Geometry check sheet. Reference: the model listing, model coordinates, mm. Coordinates: 2 decimals unless noted, no trailing zeros. Write each loop counter-clockwise with the first axis right and the second up, starting at its lowest first coordinate (ties: lowest second). Pieces come first, ordered by that corner, then holes. Notation, with made-up numbers: (-38, 19.25) - (-23, 19.25) arc R12 cw to (-23, 25.25) - close; hole circle Ø8 at (73, 5.5). An arc over 180 degrees is marked (long way). Answer as a JSON object with one key per item and string values. Group by question number.
from build123d import *

# Parameters (mm, degrees)
SKETCH_3_R          = 6.55
EXTRUDE_1_DEPTH     = 1.5
CUT_EXTRUDE_3_DEPTH = 346.626566427
EXTRUDE_2_DEPTH     = 3
CHAMFER_1_SIZE      = 4
SKETCH_8_R          = 1
SKETCH_8_R_2        = 1.6
CUT_EXTRUDE_6_DEPTH = 345.981177834
SKETCH_9_R          = 1.1
SKETCH_9_R_2        = 1.6
CUT_EXTRUDE_7_DEPTH = 345.981177834
CUT_EXTRUDE_8_DEPTH = 345.981177834
FILLET_4_R          = 50
FILLET_5_R          = 3
FILLET_6_R          = 1
EXTRUDE_3_DEPTH     = 3


with BuildPart() as part:
    # 草图3 → 凸台-拉伸1 (new, symmetric)
    # profile 1 of 2: a face of its own
    with BuildSketch(Plane(origin=(0, 0, 0), x_dir=(1, 0, 0), z_dir=(0, 1, 0))):
        with BuildLine():
            ThreePointArc((11.046281859, 5.956690113), (-6.46534327, 44.807884696), (-18.295362458, 85.748365655))
            Line((-18.295362458, 85.748365655), (-41.732882117, 195.59746049))
            Line((-41.732882117, 195.59746049), (-24.830239517, 252.12165071))
            ThreePointArc((-24.830239517, 252.12165071), (4.01455016, 296.880361934), (52.313928116, 319.29763677))
            Line((52.313928116, 319.29763677), (49.5768988, 337.088327327))
            ThreePointArc((49.5768988, 337.088327327), (-8.975981148, 310.878563044), (-45.908014731, 258.424617632))
            Line((-45.908014731, 258.424617632), (-76.290123868, 173.944647702))
            Line((-76.290123868, 173.944647702), (-14.508857835, 4.202014333))
            ThreePointArc((-14.508857835, 4.202014333), (-13.227629582, 0.452324895), (-12.09596095, -3.34517992))
            ThreePointArc((-12.09596095, -3.34517992), (-4.680454366, 11.644562977), (11.046281859, 5.956690113))
        make_face()
    # profile 2 of 2: a face of its own
    with BuildSketch(Plane(origin=(0, 0, 0), x_dir=(1, 0, 0), z_dir=(0, 1, 0))):
        with BuildLine():
            ThreePointArc((12.09596095, -3.34517992), (8.478119914, -30), (12.09596095, -56.65482008))
            ThreePointArc((12.09596095, -56.65482008), (0, -72.55), (-12.09596095, -56.65482008))
            ThreePointArc((-12.09596095, -56.65482008), (-8.478119914, -30), (-12.09596095, -3.34517992))
            ThreePointArc((-12.09596095, -3.34517992), (0, 12.55), (12.09596095, -3.34517992))
        make_face()
        with Locations(Location((0, 0, 0), (0, 0, 270))):
            Circle(SKETCH_3_R, mode=Mode.SUBTRACT)
        with Locations(Location((0, -60, 0), (0, 0, 270))):
            Circle(SKETCH_3_R, mode=Mode.SUBTRACT)
    extrude(amount=EXTRUDE_1_DEPTH, both=True)

    # 草图7 → 切除-拉伸3 (cut, through all)
    with BuildSketch(Plane(origin=(0, 1.5, 0), x_dir=(1, 0, 0), z_dir=(0, 1, 0))):
        with BuildLine():
            Line((4.497487802, -34.493479197), (8.909760465, -39.281260509))
            ThreePointArc((8.909760465, -39.281260509), (8.493926314, -31.777928612), (8.642731975, -24.264556235))
            ThreePointArc((8.642731975, -24.264556235), (7.765481215, -25.952185157), (5.921402859, -26.418055622))
            ThreePointArc((5.921402859, -26.418055622), (1.171733543, -29.743809881), (4.497487802, -34.493479197))
        make_face()
    extrude(amount=-CUT_EXTRUDE_3_DEPTH, mode=Mode.SUBTRACT)

    # 草图7<3> → 凸台-拉伸2 (add)
    with BuildSketch(Plane(origin=(0, 1.5, 0), x_dir=(1, 0, 0), z_dir=(0, 1, 0))):
        with BuildLine():
            ThreePointArc((-8.909760465, -39.281260509), (-8.493926314, -31.777928612), (-8.642731975, -24.264556235))
            ThreePointArc((-8.642731975, -24.264556235), (-8.806680236, -25.524578384), (-9.419131852, -26.637878822))
            ThreePointArc((-9.419131852, -26.637878822), (-10.758632644, -29.837669281), (-10.103316411, -33.24405769))
            ThreePointArc((-10.103316411, -33.24405769), (-9.068630527, -36.176084637), (-8.909760465, -39.281260509))
        make_face()
    extrude(amount=-EXTRUDE_2_DEPTH)

    # 倒角1
    # the kernel refuses this chamfer: 4 mm, written as the material it takes off along each edge
    with BuildSketch(Plane(origin=(49.5768988, -11.786731952, -337.088327327), x_dir=(-0.9857681497508005, 0, 0.16811054380045146), z_dir=(0, 1, 0))) as chamfer_1_piece_1:
        with BuildLine():
            Line((3.936502909, 0), (CHAMFER_1_SIZE * 0.0162625743907, CHAMFER_1_SIZE * 0.999867755593))
            Line((CHAMFER_1_SIZE * 0.0162625743907, CHAMFER_1_SIZE * 0.999867755593), (0, 0))
            ThreePointArc((0, 0), (2.023873499, -0.015992695), (3.936502909, 0))
        make_face()
    extrude(amount=23.573463904, mode=Mode.SUBTRACT)
    with BuildSketch(Plane(origin=(52.313928116, -12.013080834, -319.29763677), x_dir=(-0.15205718425393844, 0, -0.9883716976506176), z_dir=(0, 1, 0))) as chamfer_1_piece_2:
        with BuildLine():
            Line((CHAMFER_1_SIZE, 0), (-0.087315026, 4.087315025))
            ThreePointArc((-0.087315026, 4.087315025), (-0.023083391, 2.101920628), (0, 0))
            Line((0, 0), (CHAMFER_1_SIZE, 0))
        make_face()
    extrude(amount=24.026161669, mode=Mode.SUBTRACT)

    # 草图8 → 切除-拉伸6 (cut, through all)
    with BuildSketch(Plane(origin=(0, 1.5, 0), x_dir=(1, 0, 0), z_dir=(0, 1, 0))):
        with Locations((37.433203796, 321.978777823)):
            Circle(SKETCH_8_R)
        with Locations((36.505654972, 328.007845179)):
            Circle(SKETCH_8_R)
        with Locations((33.1451912, 327.490850752)):
            Circle(SKETCH_8_R)
        with Locations((34.072740024, 321.461783396)):
            Circle(SKETCH_8_R)
        with Locations(Location((44.787418503, 332.089831456, 0), (0, 0, 270))):
            Circle(SKETCH_8_R_2)
        with Locations(Location((44.787418503, 322.089831456, 0), (0, 0, 270))):
            Circle(SKETCH_8_R_2)
        with Locations((-39.768291207, 258.363013678)):
            Circle(SKETCH_8_R)
        with Locations((-40.742386095, 255.105539327)):
            Circle(SKETCH_8_R)
        with Locations((-30.091676222, 255.469378864)):
            Circle(SKETCH_8_R)
        with Locations((-31.06577111, 252.211904513)):
            Circle(SKETCH_8_R)
        with Locations((-67.294758965, 181.587091045)):
            Circle(SKETCH_8_R)
        with Locations((-65.489494047, 178.705942216)):
            Circle(SKETCH_8_R)
        with Locations((-51.956878434, 191.197471934)):
            Circle(SKETCH_8_R)
        with Locations((-50.151613516, 188.316323105)):
            Circle(SKETCH_8_R)
        with Locations((-25.036284897, 88.28804372)):
            Circle(SKETCH_8_R)
        with Locations((-25.450272298, 84.913341595)):
            Circle(SKETCH_8_R)
        with Locations((-39.031373121, 90.004873825)):
            Circle(SKETCH_8_R)
        with Locations((-39.445360522, 86.6301717)):
            Circle(SKETCH_8_R)
        Polygon((36.353597787, 328.996216876), (37.58526098, 320.990406125), (34.224797208, 320.473411699), (32.993134015, 328.47922245), align=None)
        Polygon((-40.726371898, 258.649512175), (-29.133595531, 255.182880368), (-30.107690419, 251.925406016), (-41.700466786, 255.392037824), align=None)
        Polygon((-68.142155679, 181.056130775), (-51.10948172, 191.728432204), (-49.304216802, 188.847283375), (-66.336890761, 178.174981946), align=None)
        Polygon((-40.02393257, 90.126634825), (-24.043725449, 88.16628272), (-24.45771285, 84.791580595), (-40.437919971, 86.7519327), align=None)
    extrude(amount=-CUT_EXTRUDE_6_DEPTH, mode=Mode.SUBTRACT)

    # 草图9 → 切除-拉伸7 (cut, through all)
    with BuildSketch(Plane(origin=(0, 1.5, 0), x_dir=(1, 0, 0), z_dir=(0, 1, 0))):
        with Locations(Location((-30.569466556, 243.400339284, 0), (0, 0, 270))):
            Circle(SKETCH_9_R)
        with Locations(Location((25.150787489, 314.162258091, 0), (0, 0, 270))):
            Circle(SKETCH_9_R)
        with Locations(Location((10.249770173, 305.559151733, 0), (0, 0, 270))):
            Circle(SKETCH_9_R)
        with Locations(Location((-34.866944003, 229.02912891, 0), (0, 0, 270))):
            Circle(SKETCH_9_R)
        with Locations(Location((-2.930953467, 294.499211388, 0), (0, 0, 270))):
            Circle(SKETCH_9_R)
        with Locations(Location((-39.16442145, 214.657918537, 0), (0, 0, 270))):
            Circle(SKETCH_9_R)
        with Locations(Location((-40.493555813, 175.411721209, 0), (0, 0, 270))):
            Circle(SKETCH_9_R)
        with Locations(Location((-37.363589654, 160.741911673, 0), (0, 0, 270))):
            Circle(SKETCH_9_R)
        with Locations(Location((-33.190301442, 141.182165624, 0), (0, 0, 270))):
            Circle(SKETCH_9_R)
        with Locations(Location((-33.646848365, 128, 0), (0, 0, 270))):
            Circle(SKETCH_9_R_2)
        with Locations(Location((-25.254946433, 99.197639299, 0), (0, 0, 270))):
            Circle(SKETCH_9_R_2)
        with Locations(Location((-37.131526919, 111.360979134, 0), (0, 0, 270))):
            Circle(SKETCH_9_R_2)
    extrude(amount=-CUT_EXTRUDE_7_DEPTH, mode=Mode.SUBTRACT)

    # 草图10 → 切除-拉伸8 (cut, through all)
    with BuildSketch(Plane(origin=(0, 1.5, 0), x_dir=(1, 0, 0), z_dir=(0, 1, 0))):
        Polygon((-42.197304508, 245.103074872), (-59.836896552, 196.054728732), (-47.97334255, 203.488172514), align=None)
        Polygon((-64.127048511, 169.764916812), (-48.531264313, 179.536894505), (-38.537074534, 132.695218557), (-48.388180029, 126.522731048), align=None)
    extrude(amount=-CUT_EXTRUDE_8_DEPTH, mode=Mode.SUBTRACT)

    # 圆角4
    fillet_4_edges = [part.edges().sort_by_distance(p)[0] for p in [
        (-41.732882117, 0, -195.59746049),
        (-76.290123868, 0, -173.944647702),
    ]]
    fillet(fillet_4_edges, radius=FILLET_4_R)

    # 圆角5
    fillet_5_edges = [part.edges().sort_by_distance(p)[0] for p in [
        (-48.388180029, 0, -126.522731048),
        (-64.127048511, 0, -169.764916812),
        (-48.531264313, 0, -179.536894505),
        (-38.537074534, 0, -132.695218557),
        (4.497487802, 0, 34.493479197),
        (8.909760465, 0, 39.281260509),
    ]]
    fillet(fillet_5_edges, radius=FILLET_5_R)

    # 圆角6
    fillet_6_edges = [part.edges().sort_by_distance(p)[0] for p in [
        (-42.197304508, 0, -245.103074872),
        (-47.97334255, 0, -203.488172514),
        (-59.836896552, 0, -196.054728732),
    ]]
    fillet(fillet_6_edges, radius=FILLET_6_R)

    # 草图11 → 凸台-拉伸3 (add)
    with BuildSketch(Plane(origin=(0, 1.5, 0), x_dir=(1, 0, 0), z_dir=(0, 1, 0))):
        with BuildLine():
            ThreePointArc((3.862363202, -34.328152946), (4.521977485, -34.653012522), (5.082760511, -35.12856183))
            Line((5.082760511, -35.12856183), (5.760441827, -35.863917549))
            ThreePointArc((5.760441827, -35.863917549), (4.207468493, -30.616888071), (7.413296366, -26.182284124))
            ThreePointArc((7.413296366, -26.182284124), (6.687056269, -26.42486787), (5.921402859, -26.418055622))
            ThreePointArc((5.921402859, -26.418055622), (1.241668153, -29.422934282), (3.862363202, -34.328152946))
        make_face()
        with BuildLine():
            Line((-14.508857835, 4.202014333), (-42.305901268, 80.573763491))
            ThreePointArc((-42.305901268, 80.573763491), (-22.483207982, 11.333558383), (-12.55, -60))
            ThreePointArc((-12.55, -60), (-12.435972216, -58.312073746), (-12.09596095, -56.65482008))
            ThreePointArc((-12.09596095, -56.65482008), (-10.118516623, -48.038526559), (-8.909760465, -39.281260509))
            ThreePointArc((-8.909760465, -39.281260509), (-9.068630527, -36.176084637), (-10.103316411, -33.24405769))
            ThreePointArc((-10.103316411, -33.24405769), (-10.758632644, -29.837669281), (-9.419131852, -26.637878822))
            ThreePointArc((-9.419131852, -26.637878822), (-8.806680236, -25.524578384), (-8.642731975, -24.264556235))
            ThreePointArc((-8.642731975, -24.264556235), (-10.536060501, -9.817012165), (-14.508857835, 4.202014333))
        make_face()
    extrude(amount=-EXTRUDE_3_DEPTH)


solid = part.part
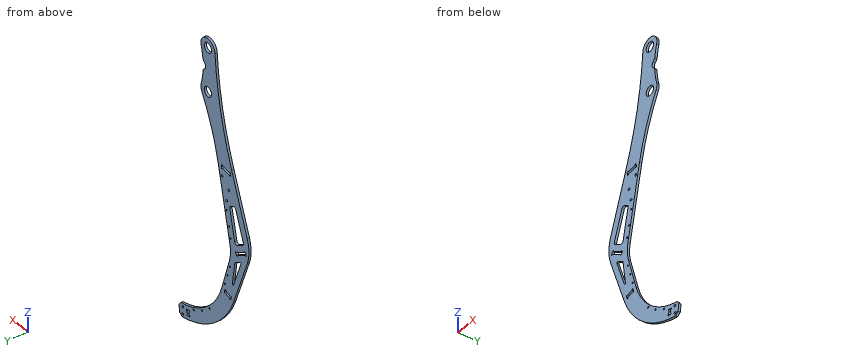
(1) Section check B-B (y = 0.05). Count the separate pieces of the cut face and the enclosed holes in it, and give its area (3 significant figures).
(2) Material ranges on L1, parallel to X at y = -0.1, z = -140.5; L2, parallel to Z at x = 5, y = -0.35; L3, parallel to X at y = -0.95, z = -100, recorded low to high. Write a range as [from, to].
(3) Section check C-C (z = -64). Record the cut outline in (x, y).
(4) Gauge pin test, flat ends, axial feed: pin 1 (1.8 mm diameter, centred on x = -40.49, z = -175.41, fed in from -Y); pin 2 (1.5 mm diameter, centred on x = 37, y = 1, fed in from +Z). Record the tip position at first contact, or that the pin passes through.
(5) Section check A-A (z = -152). Record the cut outline in (x, y).
Conclusion:
{
 "1": {"separate pieces": "1", "enclosed holes": "22", "area": "9,910 mm^2"},
 "2": {"L1": "x = [-64.12, -53.48], [-40.2, -34.05], [-32.33, -29.98]", "L2": "z = [-320.82, -297.73], [-17.79, -4.23], [4.23, 28.47], [34.85, 55.77], [64.23, 71.51]", "L3": "x = [-49.38, -26.64], [-23.87, -21.34]"},
 "3": {"outline": "(-36.59, -1.5) - (-12.8, -1.5) - (-12.8, 1.5) - (-36.59, 1.5) - close"},
 "4": {"pin 1": "passes through", "pin 2": "stops at z = -315.38"},
 "5": {"outline": "(-68.3, -1.5) - (-57.66, -1.5) - (-57.66, 1.5) - (-68.3, 1.5) - close; (-42.66, -1.5) - (-32.43, -1.5) - (-32.43, 1.5) - (-42.66, 1.5) - close"}
}
